Could you check a few things on this drawing? It's one solid part, dimensions in mm from its lowest x, y, z. Coordinates: 2 decimals unless noted, no trailing zeros. Order: outer loops, then holes, each group sorted by start corner. A loop starts at its lowest first (then second) coordinate and runs counter-clockwise, first axis right, second up. Notation, with made-up numbers: M 47,64 L 68,64 A27 ccw 68,84 Z; hole C -10,53 d10. An arc over 180 degrees is marked long. Answer as CSV lines item,"result". Start each with the question number.
1. If we section it at B-B (x = 30.5): List the corners of the cut face in (y, z) for me (1 decimal).
2. I need wall thicknesses on line 1 along Z through (x, y) = (51.5, 2.35) (1 decimal); line 2 along Y through (x, z) = (60.5, 4.5). Which ranges of each line are inside material? Lowest first, please. Write a range as from..to.
3. If we section it at A-A (y = 2.15): List the corners of the cut face in (x, z) for me (1 decimal), plus the area to 3 significant figures.
4. Will these pins go through, and if not, where does the flat tip stop? pin 1 (0.5 mm diameter, centred on x = 22, y = 2, fed in from -Z); pin 2 (1.6 mm diameter, centred on x = 30, z = 34.5, fed in from +Y).
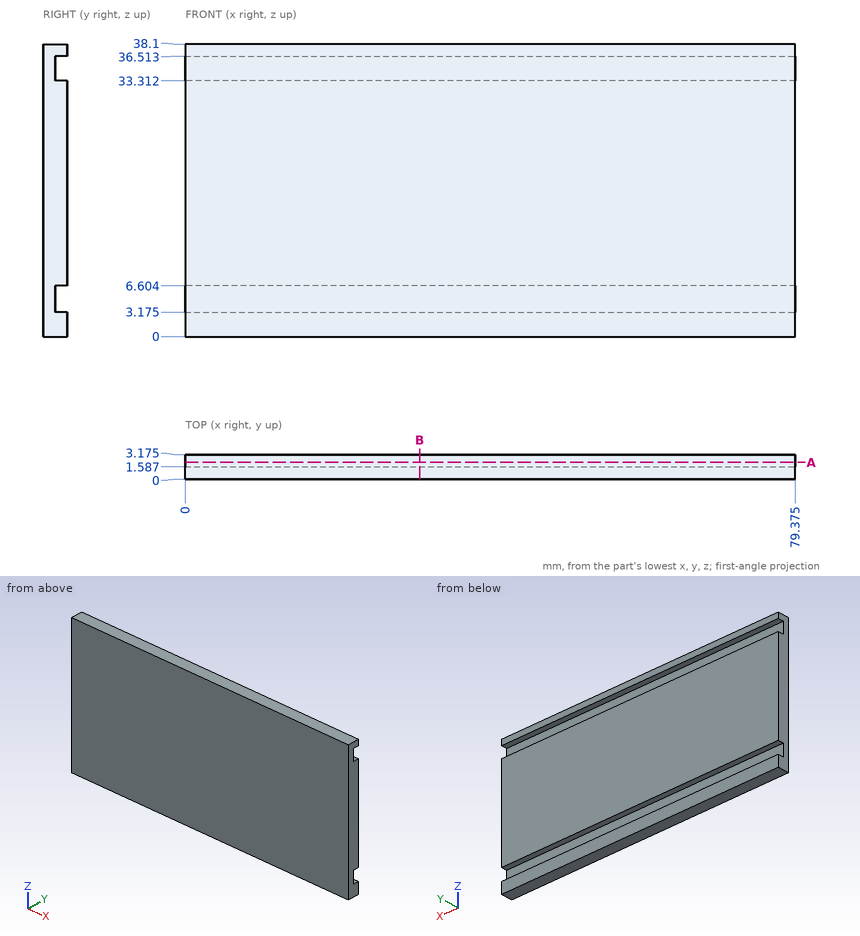
Solved:
1,outline,"M 0,0 L 3.2,0 L 3.2,3.2 L 1.6,3.2 L 1.6,6.6 L 3.2,6.6 L 3.2,33.3 L 1.6,33.3 L 1.6,36.5 L 3.2,36.5 L 3.2,38.1 L 0,38.1 Z"
2,line 1,"0..3.2, 6.6..33.3, 36.5..38.1"
2,line 2,"0..1.59"
3,outline,"M 0,0 L 79.4,0 L 79.4,3.2 L 0,3.2 Z; M 0,6.6 L 79.4,6.6 L 79.4,33.3 L 0,33.3 Z; M 0,36.5 L 79.4,36.5 L 79.4,38.1 L 0,38.1 Z"
3,area,"2,500 mm²"
4,pin 1,"z = 0"
4,pin 2,"y = 1.59"
